from build123d import *

# Parameters (mm, degrees)
SKETCH2_W                        = 127
SKETCH2_H                        = 127
HOUSING_DEPTH                    = 39.5
SKETCH4_OUTSIDE_W                = 165.78
SKETCH4_OUTSIDE_H                = 165.78
SKETCH4_OUTSIDE_R                = 45.974
CUT_EXTRUDE2_DEPTH               = 4.698
MOUNTING_POCKETS_DEPTH           = 24.384
ENG_METRIC_SLOT_VERTICAL_REACH   = 129
ENG_METRIC_SLOT_HORIZONTAL_DEPTH = 40.5
FILLET3_R                        = 0.508
SKETCH213_W                      = 57.15
SKETCH213_H                      = 57.15
EXTRUDE1_DEPTH                   = 26.924
SKETCH214_R                      = 23.8125
CUT_EXTRUDE3_DEPTH               = 5
SKETCH215_R                      = 3.175
CUT_EXTRUDE4_DEPTH               = 21.924
CUT_EXTRUDE5_REACH               = 131.159
SKETCH216_W                      = 42.545
SKETCH216_H                      = 3.048
F_8_32_TAPPED_HOLE1_D            = 3.4544
F_8_32_TAPPED_HOLE1_DEPTH        = 10.7086
F_8_32_TAPPED_HOLE1_TIP          = 1.037806461
SKETCH241_R                      = 45.974
CUT_EXTRUDE7_DEPTH               = 4.698
SKETCH3_R                        = 22.5
CUT_EXTRUDE8_DEPTH               = 49.26


with BuildPart() as part:
    # Sketch2 → HOUSING (new body)
    with BuildSketch(Plane.XY):
        Rectangle(SKETCH2_W, SKETCH2_H)
    extrude(amount=HOUSING_DEPTH)

    # Sketch4 outside → Cut-Extrude2 (cut)
    with BuildSketch(Plane.XY.offset(39.5)):
        Rectangle(SKETCH4_OUTSIDE_W, SKETCH4_OUTSIDE_H)
        Circle(SKETCH4_OUTSIDE_R, mode=Mode.SUBTRACT)
    extrude(amount=-CUT_EXTRUDE2_DEPTH, mode=Mode.SUBTRACT)

    # Sketch8 → MOUNTING POCKETS (cut)
    with BuildSketch(Plane.XY.offset(34.802)):
        with BuildLine():
            Line((3.048, -63.5), (3.048, -57.528018122))
            ThreePointArc((3.048, -57.528018122), (4.194729662, -53.888172274), (7.220748912, -51.562946647))
            Line((7.220748912, -51.562946647), (45.320748912, -37.656446647))
            ThreePointArc((45.320748912, -37.656446647), (51.137845848, -38.418247784), (53.848, -43.621518122))
            Line((53.848, -43.621518122), (53.848, -63.5))
            Line((53.848, -63.5), (3.048, -63.5))
        make_face()
        with BuildLine():
            Line((3.048, 63.5), (53.848, 63.5))
            Line((53.848, 63.5), (53.848, 43.621518122))
            ThreePointArc((53.848, 43.621518122), (51.137845848, 38.418247784), (45.320748912, 37.656446647))
            Line((45.320748912, 37.656446647), (7.220748912, 51.562946647))
            ThreePointArc((7.220748912, 51.562946647), (4.194729662, 53.888172274), (3.048, 57.528018122))
            Line((3.048, 57.528018122), (3.048, 63.5))
        make_face()
    extrude(amount=-MOUNTING_POCKETS_DEPTH, mode=Mode.SUBTRACT)

    # Sketch21 → ENG_METRIC SLOT VERTICAL (cut, up to next)
    with BuildSketch(Plane(origin=(63.5, -23.646142673, 1.166551585), x_dir=(0, 0, -1), z_dir=(1, 0, 0)), mode=Mode.PRIVATE) as eng_metric_slot_vertical_sk1:
        with BuildLine():
            Line((-20.641506099, 75.242113831), (-21.041506099, 76.042113831))
            ThreePointArc((-21.041506099, 76.042113831), (-25.829419573, 77.63808499), (-27.425390732, 72.850171515))
            Line((-27.425390732, 72.850171515), (-27.025390732, 72.050171515))
            ThreePointArc((-27.025390732, 72.050171515), (-22.237477257, 70.454200357), (-20.641506099, 75.242113831))
        make_face()
    eng_metric_slot_vertical_tool1 = extrude(eng_metric_slot_vertical_sk1.sketch, amount=-ENG_METRIC_SLOT_VERTICAL_REACH, mode=Mode.PRIVATE) & part.part
    add(eng_metric_slot_vertical_tool1.solids().sort_by_distance((63.5, 50.4, 25.2))[0], mode=Mode.SUBTRACT)
    # Sketch21 → ENG_METRIC SLOT VERTICAL (cut, up to next)
    with BuildSketch(Plane(origin=(63.5, -23.646142673, 1.166551585), x_dir=(0, 0, -1), z_dir=(1, 0, 0)), mode=Mode.PRIVATE) as eng_metric_slot_vertical_sk2:
        with BuildLine():
            Line((-27.025390732, -24.757886169), (-27.425390732, -25.557886169))
            ThreePointArc((-27.425390732, -25.557886169), (-25.829419573, -30.345799643), (-21.041506099, -28.749828485))
            Line((-21.041506099, -28.749828485), (-20.641506099, -27.949828485))
            ThreePointArc((-20.641506099, -27.949828485), (-22.237477257, -23.16191501), (-27.025390732, -24.757886169))
        make_face()
    eng_metric_slot_vertical_tool2 = extrude(eng_metric_slot_vertical_sk2.sketch, amount=-ENG_METRIC_SLOT_VERTICAL_REACH, mode=Mode.PRIVATE) & part.part
    add(eng_metric_slot_vertical_tool2.solids().sort_by_distance((63.5, -50.4, 25.2))[0], mode=Mode.SUBTRACT)

    # Sketch212 → ENG_METRIC SLOT HORIZONTAL (cut, through all)
    with BuildSketch(Plane(origin=(34.062086582, -104.655987826, 0), x_dir=(-1, 0, 0), z_dir=(0, 0, -1))):
        with BuildLine():
            Line((12.254028899, 156.251958985), (11.854028899, 157.051958985))
            ThreePointArc((11.854028899, 157.051958985), (7.066115424, 158.647930143), (5.470144266, 153.860016668))
            Line((5.470144266, 153.860016668), (5.870144266, 153.060016668))
            ThreePointArc((5.870144266, 153.060016668), (10.658057741, 151.46404551), (12.254028899, 156.251958985))
        make_face()
        with BuildLine():
            Line((5.870144266, 56.251958985), (5.470144266, 55.451958985))
            ThreePointArc((5.470144266, 55.451958985), (7.066115424, 50.66404551), (11.854028899, 52.260016668))
            Line((11.854028899, 52.260016668), (12.254028899, 53.060016668))
            ThreePointArc((12.254028899, 53.060016668), (10.658057741, 57.847930143), (5.870144266, 56.251958985))
        make_face()
    extrude(amount=-ENG_METRIC_SLOT_HORIZONTAL_DEPTH, mode=Mode.SUBTRACT)

    # Fillet3
    fillet3_edges = [part.edges().sort_by_distance(p)[0] for p in [
        (3.048, -60.514009061, 10.418),
        (4.194729662, -53.888172274, 10.418),
        (26.270748912, -44.609696647, 10.418),
        (51.137845848, -38.418247784, 10.418),
        (53.848, -53.560759061, 10.418),
        (51.137845848, 38.418247784, 10.418),
        (26.270748912, 44.609696647, 10.418),
        (4.194729662, 53.888172274, 10.418),
        (3.048, 60.514009061, 10.418),
        (53.848, 53.560759061, 10.418),
    ]]
    fillet(fillet3_edges, radius=FILLET3_R)

    # Sketch213 → Extrude1 (add)
    with BuildSketch(Plane.XZ.offset(63.5)):
        with Locations((-37.084, 30.48)):
            Rectangle(SKETCH213_W, SKETCH213_H)
    extrude(amount=EXTRUDE1_DEPTH)

    # Sketch214 → Cut-Extrude3 (cut)
    with BuildSketch(Plane.XZ.offset(90.424)):
        with Locations((-37.084, 30.48)):
            Circle(SKETCH214_R)
    extrude(amount=-CUT_EXTRUDE3_DEPTH, mode=Mode.SUBTRACT)

    # Sketch215 → Cut-Extrude4 (cut)
    with BuildSketch(Plane.XZ.offset(85.424)):
        with Locations((-37.084, 30.48)):
            Circle(SKETCH215_R)
    extrude(amount=-CUT_EXTRUDE4_DEPTH, mode=Mode.SUBTRACT)

    # Sketch216 → Cut-Extrude5 (cut, up to next)
    with BuildSketch(Plane.ZY.offset(65.659), mode=Mode.PRIVATE) as cut_extrude5_sk1:
        with Locations((37.7825, -65.024)):
            Rectangle(SKETCH216_W, SKETCH216_H)
    cut_extrude5_tool1 = extrude(cut_extrude5_sk1.sketch, amount=-CUT_EXTRUDE5_REACH, mode=Mode.PRIVATE) & part.part
    add(cut_extrude5_tool1.solids().sort_by_distance((-65.659, -65.024, 37.7825))[0], mode=Mode.SUBTRACT)

    # #8-32 Tapped Hole1
    with Locations(Plane.XZ.offset(90.424)):
        with Locations((-60.706, 6.858), (-60.706, 54.102), (-13.462, 54.102), (-13.462, 6.858)):
            Hole(F_8_32_TAPPED_HOLE1_D / 2, depth=F_8_32_TAPPED_HOLE1_DEPTH)
            with Locations((0, 0, -(F_8_32_TAPPED_HOLE1_DEPTH + F_8_32_TAPPED_HOLE1_TIP / 2))):  # 118° drill point
                Cone(0, F_8_32_TAPPED_HOLE1_D / 2, F_8_32_TAPPED_HOLE1_TIP, mode=Mode.SUBTRACT)

    # Sketch241 → Cut-Extrude7 (cut)
    with BuildSketch(Plane.XY.offset(39.5)):
        Circle(SKETCH241_R)
    extrude(amount=-CUT_EXTRUDE7_DEPTH, mode=Mode.SUBTRACT)

    # Sketch3 → Cut-Extrude8 (cut, through all)
    with BuildSketch(Plane.XY.offset(48.26)):
        Circle(SKETCH3_R)
    extrude(amount=-CUT_EXTRUDE8_DEPTH, mode=Mode.SUBTRACT)


solid = part.part
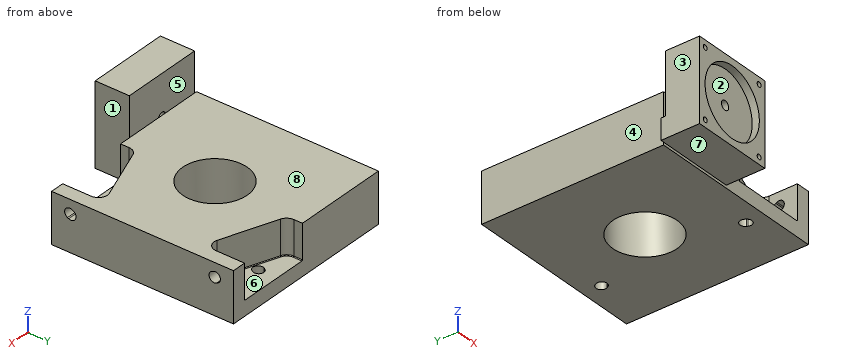
For this review, take the finished solid that the model builds, in its own axes (mm). Face numbers are marked on the shaded views. A direction names the side the tool comes from. Coordinates: 2 decimals unless noted, no trailing zeros. Order: outer loops, then holes, each group sorted by start corner. A loop starts at its lowest first (then second) coordinate and runs counter-clockwise, first axis right, second up. Notation, with made-up numbers: (-25.5, -0.75) -> (-13.5, -0.75) arc R16 ccw to (-13.5, 14.25) -> close; hole circle Ø1 at (-32, 16). An arc over 180 degrees is marked (long way). Return JSON: item names as keys, results as strings.
1. For line 1 (Y direction, x = 0, z = 16); line 2 (Y direction, x = -15.5, z = 33.5); line 3 (Y direction, x = -46, z = 22), list the stretches that pass through material, from the lowest coordinate up. Write a range as from..to.
Answer block:
{"line 1": "-63.5..-22.5, 22.5..63.5", "line 2": "-85.42..-66.55, -63.5..-16.31, 16.31..63.5", "line 3": "-85.42..-66.55, -63.5..63.5"}
2. Machinability: for the marked faces 4, 5, 6, 7 and 8, which of the approach directions +Z, -Z, +X, -X, +Y, -Y give a long, thin tool a straight path to every point of the face, cutting with its end or side? Answer none if there is none.
Answer block:
{"face 4": "+Z, -Z, -X, +Y", "face 5": "+Z, +X, -X", "face 6": "+Z, +Y", "face 7": "-Z, +X, -X, -Y", "face 8": "+Z, +X, -X, +Y"}
3. We need section C-C on x = -51. Write out the cut boundary in (y, z) (3 decimals).
Answer block:
{"outline": "(-90.424, 1.905) -> (-63.5, 1.905) -> (-63.5, 0) -> (63.5, 0) -> (63.5, 34.802) -> (-63.5, 34.802) -> (-63.5, 16.51) -> (-66.548, 16.51) -> (-66.548, 59.055) -> (-90.424, 59.055) -> (-90.424, 49.803) -> (-85.424, 49.803) -> (-85.424, 11.157) -> (-90.424, 11.157) -> close"}
4. We need section A-A on x = 0. Write out the cut boundary in (y, z), and give its area (3 significant figures).
Answer block:
{"outline": "(-63.5, 0) -> (-22.5, 0) -> (-22.5, 34.8) -> (-63.5, 34.8) -> close; (22.5, 0) -> (63.5, 0) -> (63.5, 34.8) -> (22.5, 34.8) -> close", "area": "2,850 mm²"}
5. We need section B-B on z = 37.5. Write out the cut boundary in (x, y), and give its area (3 significant figures).
Answer block:
{"outline": "(-65.66, -90.42) -> (-59.84, -90.42) -> (-59.84, -85.42) -> (-14.33, -85.42) -> (-14.33, -90.42) -> (-8.51, -90.42) -> (-8.51, -66.55) -> (-65.66, -66.55) -> close", "area": "1,140 mm²"}
6. We need section D-D on y = -35. Write out the cut boundary in (x, z), and give its area (3 significant figures).
Answer block:
{"outline": "(-63.5, 0) -> (63.5, 0) -> (63.5, 34.8) -> (-63.5, 34.8) -> close", "area": "4,420 mm²"}
7. For pin 1 Ø21.5 at (x, y) = (-25, -75) entering from -Z (3 decimals); pin 2 Ø17.5 at (x, z) = (10.5, 24.5) entering from -Y; pin 3 Ø10 at (x, y) = (40.5, -45) entering from -Z; pin 4 Ø4.5 at (x, z) = (-13.462, 54.102) entering from +Y, all flat-tipped, find the tip position at first contact; note any pin that passes through.
Answer block:
{"pin 1": "z = 1.905", "pin 2": "y = -63.5", "pin 3": "z = 0", "pin 4": "y = -66.55"}
8. The part is to be moulded in two halves that separate along X. For the marked faces 1, 2 and 3, say which applies: +X half, -X half, draft (parallel to the pull), parting line (faces both ways), or undercut.
Answer block:
{"face 1": "+X half", "face 2": "undercut", "face 3": "-X half"}
